Source: CAD feature listing. Evaluate the final solid. Frame: model axes, mm. A direction names the side the tool comes from. Coordinates: 2 decimals unless noted, no trailing zeros. Order: outer loops, then holes, each group sorted by start corner. A loop starts at its lowest first (then second) coordinate and runs counter-clockwise, first axis right, second up. Notation, with made-up numbers: (22.25, 89) -> (61.25, 89) arc R28 ccw to (61.25, 122) -> close; hole circle Ø5 at (5, 61.25). An arc over 180 degrees is marked (long way). Write item = value, one per line. Start each with the question number.
Item 1: Contact query for flat-ended pins moving along their axis: pin 1 (3 mm diameter, centred on x = -1097, z = -11.5, fed in from -Y); pin 2 (6 mm diameter, centred on x = -1319, z = -9, fed in from +Y); pin 3 (8 mm diameter, centred on x = -800, y = 165.5, fed in from +Z). Output: stop coordinate, or through.
Item 2: Ray query, line 1 along Z through (x, y) = (-93.5, 110); line 2 along Z through (x, y) = (-1450.5, 167.5); line 3 along Y through (x, z) = (-298, -5). Return the intervals inside material, ascending. Write a range as [from, to].
Item 3: Set-up query: faces 1 (the flat face through (-2390, 90, 7)), 2 (the flat face through (-1178, 155, 10)), 3 (the flat face through (-1202, 94, 0)). Return all of +Z, -Z, +X, -X, +Y, -Y with unobstructed straight access to the full face (end or side cutting, diameter ignored); none if empty.
Item 4: Section query A-A (y = 149.5). Output: boundary loops of the cut face in (x, z), then the cut area to 3 significant figures.
Item 5: Section query B-B (x = -718). Output: boundary loops of the cut face in (y, z).
```python
from build123d import *

# Parameters (mm, degrees)
F1_DEPTH    = 2390
F3_DEPTH    = 20
F5_DEPTH    = 10
F6_T1_DEPTH = 216.618628623
F6_T3_DEPTH = 142.4030805268
F6_T5_DEPTH = 100.344113211
F6_T7_DEPTH = 68.9770272469


# Not quite as in the source:
# - a fillet or chamfer that OpenCascade refuses, or shapes differently, is made with other operations: its cross-section is extruded or revolved along the edge and cut away or added


with BuildPart() as f1:
    # F0 (on Right) → F1 (new body)
    with BuildSketch(Plane.YZ):
        with BuildLine():
            Line((0, -19.8239199817), (0, 0))
            Line((0, 0), (190, 0))
            Line((190, 0), (190, 10))
            Line((190, 10), (120, 10))
            Line((120, 10), (120, 19.1649627105))
            ThreePointArc((120, 19.1649627105), (118.4117029432, 22.8201348033), (114.655886789, 24.1531072651))
            Line((114.655886789, 24.1531072651), (-2.4688205766, 16.0731170599))
            ThreePointArc((-2.4688205766, 16.0731170599), (-5.8715951564, 14.3956872139), (-7.1172645938, 10.8122596114))
            Line((-7.1172645938, 10.8122596114), (-6.3410848379, -15.7684031874))
            ThreePointArc((-6.3410848379, -15.7684031874), (-4.7310556973, -18.6708970152), (-1.618628623, -19.8239199817))
            Line((-1.618628623, -19.8239199817), (0, -19.8239199817))
        make_face()
    extrude(amount=-F1_DEPTH)

    # F2 (on face) → F3 (join)
    with BuildSketch(Plane.YZ):
        with BuildLine():
            ThreePointArc((-6.3410848379, -15.7684031874), (-4.7310556973, -18.6708970152), (-1.618628623, -19.8239199817))
            Line((-1.618628623, -19.8239199817), (0, -19.8239199817))
            Line((0, -19.8239199817), (0, 0))
            Line((0, 0), (190, 0))
            Line((190, 0), (190, 10))
            Line((190, 10), (120, 10))
            Line((120, 10), (120, 19.1649627105))
            ThreePointArc((120, 19.1649627105), (118.6551720927, 22.5766656537), (115.344113211, 24.1531072651))
            Line((115.344113211, 24.1531072651), (114.655886789, 24.1531072651))
            Line((114.655886789, 24.1531072651), (-2.4688205766, 16.0731170599))
            ThreePointArc((-2.4688205766, 16.0731170599), (-5.8715951564, 14.3956872139), (-7.1172645938, 10.8122596114))
            Line((-7.1172645938, 10.8122596114), (-6.3410848379, -15.7684031874))
        make_face()
        with BuildLine():
            Line((120, 10), (190, 10))
            Line((190, 10), (190, 24.1531072651))
            Line((190, 24.1531072651), (115.344113211, 24.1531072651))
            ThreePointArc((115.344113211, 24.1531072651), (118.6551720927, 22.5766656537), (120, 19.1649627105))
            Line((120, 19.1649627105), (120, 10))
        make_face()
    extrude(amount=F3_DEPTH)

    # F4 (on face) → F5 (join)
    with BuildSketch(Plane.YZ.offset(20)):
        with BuildLine():
            Line((190, -19.8239199817), (190, 0))
            Line((190, 0), (190, 24.1531072651))
            Line((190, 24.1531072651), (114.655886789, 24.1531072651))
            Line((114.655886789, 24.1531072651), (-2.4688205766, 16.0731170599))
            ThreePointArc((-2.4688205766, 16.0731170599), (-5.8715951564, 14.3956872139), (-7.1172645938, 10.8122596114))
            Line((-7.1172645938, 10.8122596114), (-6.3410848379, -15.7684031874))
            ThreePointArc((-6.3410848379, -15.7684031874), (-4.7310556973, -18.6708970152), (-1.618628623, -19.8239199817))
            Line((-1.618628623, -19.8239199817), (0, -19.8239199817))
            Line((0, -19.8239199817), (190, -19.8239199817))
        make_face()
    extrude(amount=F5_DEPTH)

    # F6: fillet of radius 5 on 4 edges, made by hand

    # F6_s2 → F6_t1 (cut)
    with BuildSketch(Plane.XZ.offset(-202.5)):
        with BuildLine():
            ThreePointArc((30, -14.8239199817), (28.5355339059, -18.3594538877), (25, -19.8239199817))
            Line((25, -19.8239199817), (30, -19.8239199817))
            Line((30, -19.8239199817), (30, -14.8239199817))
        make_face()
    extrude(amount=F6_T1_DEPTH, mode=Mode.SUBTRACT)

    # F6_s4 → F6_t3 (cut)
    with BuildSketch(Plane(origin=(0, 128.2415133818, 8.8468965716), x_dir=(1, 0, 0), z_dir=(0, -0.9976289109, -0.0688226422))):
        with BuildLine():
            ThreePointArc((25, 16.2049170229), (28.5355339059, 14.7404509288), (30, 11.2049170229))
            Line((30, 11.2049170229), (30, 16.2049170229))
            Line((30, 16.2049170229), (25, 16.2049170229))
        make_face()
    extrude(amount=F6_T3_DEPTH, mode=Mode.SUBTRACT)

    # F6_s6 → F6_t5 (cut)
    with BuildSketch(Plane.XZ.offset(-202.5)):
        with BuildLine():
            ThreePointArc((25, 24.1531072651), (28.5355339059, 22.6886411711), (30, 19.1531072651))
            Line((30, 19.1531072651), (30, 24.1531072651))
            Line((30, 24.1531072651), (25, 24.1531072651))
        make_face()
    extrude(amount=F6_T5_DEPTH, mode=Mode.SUBTRACT)

    # F6_s8 → F6_t7 (cut)
    with BuildSketch(Plane.XY.offset(-32.3239199817)):
        with BuildLine():
            ThreePointArc((25, 190), (28.5355339059, 188.5355339059), (30, 185))
            Line((30, 185), (30, 190))
            Line((30, 190), (25, 190))
        make_face()
    extrude(amount=F6_T7_DEPTH, mode=Mode.SUBTRACT)


solid = f1.part
```
Computed:
q1.pin_1 = -6.51
q1.pin_2 = 0
q1.pin_3 = 10
q2.line_1 = [0, 23.83]
q2.line_2 = [0, 10]
q2.line_3 = [-6.66, 0]
q3.face_1 = +Z, -Z, -X, +Y, -Y
q3.face_2 = +Z, -X, +Y
q3.face_3 = -Z, -X, +Y
q4.outline = (-2390, 0) -> (20, 0) -> (20, -19.82) -> (25, -19.82) arc R5 ccw to (30, -14.82) -> (30, 19.15) arc R5 ccw to (25, 24.15) -> (0, 24.15) -> (0, 10) -> (-2390, 10) -> close
q4.area = 24,800 mm^2
q5.outline = (-7.12, 10.81) -> (-6.34, -15.77) arc R4.78 ccw to (-1.62, -19.82) -> (0, -19.82) -> (0, 0) -> (190, 0) -> (190, 10) -> (120, 10) -> (120, 19.16) arc R5 ccw to (114.66, 24.15) -> (-2.47, 16.07) arc R5 ccw to start
